The model under review builds one solid part; all positions refer to its coordinate system, in mm. Face numbers are marked on the shaded views. A direction names the side the tool comes from. Coordinates: 2 decimals unless noted, no trailing zeros. Order: outer loops, then holes, each group sorted by start corner. A loop starts at its lowest first (then second) coordinate and runs counter-clockwise, first axis right, second up. Notation, with made-up numbers: (85, 83.5) -> (89, 83.5) arc R24 ccw to (89, 99.5) -> close; hole circle Ø8 at (3.25, -9.5). An arc over 180 degrees is marked (long way). Answer as CSV lines item,"result". Start each with the question number.
from build123d import *

# Parameters (mm, degrees)
F0_W     = 15.5
F0_H     = 8.1
F0_W_2   = 10.9
F0_H_2   = 8.3
F0_R     = 4
F1_DEPTH = 15
F2_W     = 11.035934
F2_H     = 3.300466
F2_W_2   = 12.273613
F2_H_2   = 3.464567
F2_W_3   = 14.223677
F2_H_3   = 3.989566
F3_DEPTH = 12.5
F4_R     = 2.25
F5_DEPTH = 25
F6_DEPTH = 2
F7_R     = 5
F8_R     = 3
F9_SIZE2 = 3.732051
F9_SIZE  = 1


with BuildPart() as f1:
    # F0 (on Right) → F1 (new body)
    with BuildSketch(Plane.YZ):
        Polygon((42.32502, 23.932349), (42.32502, 35.553029), (-49.718533, 35.553029), (-49.718533, 23.932349), (4.384954, 23.932349), (4.384954, 24.508461), (4.384954, 33.808461), (25.584954, 33.808461), (25.584954, 24.508461), (25.584954, 23.932349), align=None)
        with Locations((-39.568292, 29.758461)):
            Rectangle(F0_W, F0_H, mode=Mode.SUBTRACT)
        with Locations((-14.972494, 29.658461)):
            Rectangle(F0_W_2, F0_H_2, mode=Mode.SUBTRACT)
        with Locations((36.776925, 29.86361)):
            Circle(F0_R, mode=Mode.SUBTRACT)
        Polygon((4.384954, 24.508461), (4.384954, 23.932349), (6.113291, 23.932349), align=None)
        Polygon((23.856617, 23.932349), (25.584954, 23.932349), (25.584954, 24.508461), align=None)
    extrude(amount=-F1_DEPTH)

    # F2 (on face) → F3 (cut)
    with BuildSketch(Plane(origin=(-15, 0, 0), x_dir=(0, -1, 0), z_dir=(-1, 0, 0))):
        with Locations((-29.337391, 28.200673)):
            Rectangle(F2_W, F2_H)
        with Locations((-0.870865, 27.251326)):
            Rectangle(F2_W_2, F2_H_2)
        with Locations((25.624747, 27.518563)):
            Rectangle(F2_W_3, F2_H_3)
    extrude(amount=-F3_DEPTH, mode=Mode.SUBTRACT)

    # F4 (on face) → F5 (cut)
    with BuildSketch(Plane.XY.offset(35.553029)):
        with Locations((-10.227251, 29.789448)):
            Circle(F4_R)
        with Locations((-10.573186, 2.008814)):
            Circle(F4_R)
        with Locations((-10.457753, -26.231565)):
            Circle(F4_R)
    extrude(amount=-F5_DEPTH, mode=Mode.SUBTRACT)

    # F4 (on face) → F6 (cut)
    with BuildSketch(Plane.XY.offset(35.553029)):
        Polygon((-11.870602, 26.94308), (-8.5839, 26.94308), (-6.940549, 29.789448), (-8.5839, 32.635815), (-11.870602, 32.635815), (-13.513953, 29.789448), align=None)
        with Locations((-10.227251, 29.789448)):
            Circle(F4_R, mode=Mode.SUBTRACT)
        Polygon((-12.268482, -29.367838), (-8.647025, -29.367838), (-6.836297, -26.231565), (-8.647025, -23.095291), (-12.268482, -23.095291), (-14.07921, -26.231565), align=None)
        with Locations((-10.457753, -26.231565)):
            Circle(F4_R, mode=Mode.SUBTRACT)
        Polygon((-8.576097, 4.384954), (-12.570275, 4.384954), (-13.94214, 2.008814), (-12.257663, -0.908786), (-8.888709, -0.908786), (-7.204232, 2.008814), align=None)
        with Locations((-10.573186, 2.008814)):
            Circle(F4_R, mode=Mode.SUBTRACT)
    extrude(amount=-F6_DEPTH, mode=Mode.SUBTRACT)

    # F7
    f7_edges = [f1.edges().sort_by_distance(p)[0] for p in [
        (-7.5, 42.32502, 23.932349),
        (-7.5, 42.32502, 35.553029),
    ]]
    fillet(f7_edges, radius=F7_R)

    # F8
    f8_edges = [f1.edges().sort_by_distance(p)[0] for p in [
        (-7.5, -49.718533, 35.553029),
        (-7.5, -49.718533, 23.932349),
    ]]
    fillet(f8_edges, radius=F8_R)

    # F9
    f9_edges = [f1.edges().sort_by_distance(p)[0] for p in [
        (0, -4.696756, 35.553029),
    ]]
    chamfer(f9_edges, length=F9_SIZE, length2=F9_SIZE2)


solid = f1.part
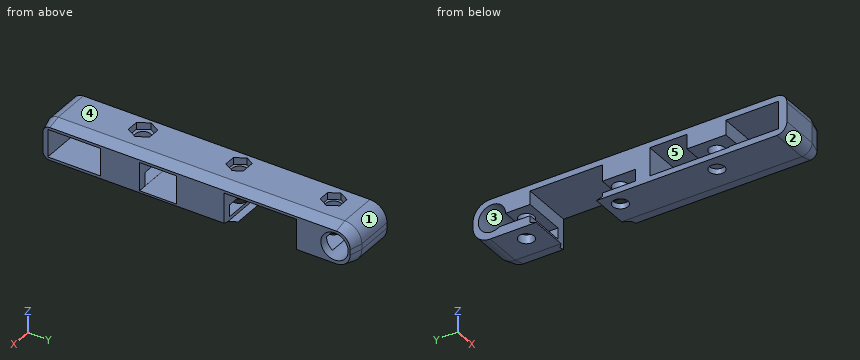
1) Tool access review of the marked faces 4 and 5: name each direction out of +Z, -Z, +X, -X, +Y, -Y from which nothing blocks a thin tool from reaching the whole face with its end or side.
2) Mouldability with a two-part tool opening along Z and no side actions: class the marked faces 1, 2 and 3 as released by +Z, released by -Z, zero draft, split by the parting line, or undercut.
3) Wall thickness on L1, parallel to Z at x = -8.5, y = -31.5; L2, parallel to Y at x = -5.25, z = 33; L3, parallel to Z at x = -13, y = -34.5: over which ranges is each line inside the solid? List them lowest first. Write a range as [from, to].
4) Insertion check: pin 1 Ø1 at (x, z) = (-10.5, 34.5) entering from +Y; pin 2 Ø2.5 at (x, y) = (-12, 2) entering from +Z; pin 3 Ø1.9 at (x, z) = (-11, 34.5) entering from -Y. Each pin has a flat end and moves straight along its axis. Give the tip position at first contact, or say it passes through.
5) Consider section B-B (y = -4). Give the boundary of the cut face in (x, z), plus the area to 3 significant figures.
6) Consider section C-C (z = 31.5). Count the separate pieces of the cut face and the enclosed holes in it, plus the area to 3 significant figures.
7) Consider section A-A (y = -39.5). Give the boundary of the cut face in (x, z).
Result:
1,face 4,"+Z, +X, -X, +Y, -Y"
1,face 5,"+X, -X"
2,face 1,"released by +Z"
2,face 2,"released by -Z"
2,face 3,"undercut"
3,L1,"[23.93, 25.52], [29.51, 35.55]"
3,L2,"[-49.69, -47.32], [-31.82, -20.42], [-9.52, 4.38], [25.58, 34.29], [39.26, 41.69]"
3,L3,"[23.93, 25.71], [33.81, 35.55]"
4,pin 1,"y = 40.95"
4,pin 2,"z = 33.55"
4,pin 3,"y = -49.55"
5,outline,"(-15, 23.93) -> (-3.73, 23.93) -> (0, 24.93) -> (0, 34.55) -> (-3.73, 35.55) -> (-15, 35.55) -> (-15, 28.98) -> (-2.5, 28.98) -> (-2.5, 25.52) -> (-15, 25.52) -> close"
5,area,"127 mm2"
6,separate pieces,"5"
6,enclosed holes,"3"
6,area,"504 mm2"
7,outline,"(-15, 23.93) -> (-3.73, 23.93) -> (0, 24.93) -> (0, 25.71) -> (-15, 25.71) -> close; (-15, 33.81) -> (0, 33.81) -> (0, 34.55) -> (-3.73, 35.55) -> (-15, 35.55) -> close"
